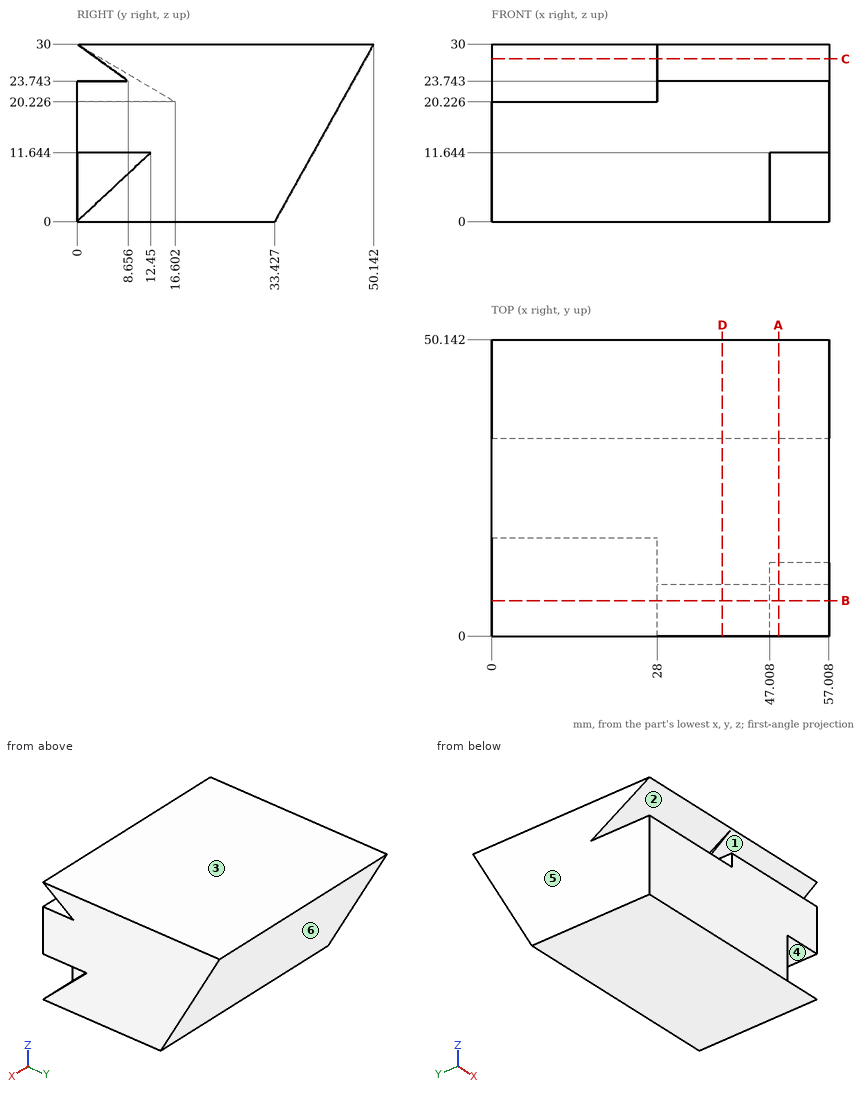
Verification items for this drawing (mm, ordinates from the low corner). A direction names the side the tool comes from. Give positions to 0.01 mm unless a question says otherwise; leave off trailing zeros. Loops run counter-clockwise (first coordinate to the right, second up) from the corner with the lowest first, then second, coordinate; pieces in that order, holes last. Notation, with made-up numbers: M -16.75,28 L 2.25,28 A14 ccw 2.25,42 Z; hole C -11,-10 d7. An arc over 180 degrees is marked long. Return JSON: item names as keys, results as strings. Group by question number.
1. Cross-section at A-A on x = 48.5. Record the boundary of the cut face in (y, z).
2. Tool access check on the marked faces 1, 2 and 3. Record the directions out of +Z, -Z, +X, -X, +Y, -Y that give a thin tool (end or side, any length) a straight path to the whole face; none if there is none.
3. Thickness scan on L1, parallel to Z at x = 8, y = 8.5 (1 decimal); L2, parallel to X at y = 10, z = 11.5; L3, parallel to Z at x = 5.5, y = 10.5 (1 decimal). Record the ranges inside material, lowest first.
4. Cross-section at D-D on x = 39. Record the boundary of the cut face in (y, z), plus the area to 3 significant figures.
5. Cross-section at C-C on z = 27.5. Record the boundary of the cut face in (x, y), plus the area to 3 significant figures.
6. Mould release check, pull along Z, two halves, no side actions. Record for the marked faces 4, 5 and 6: released by +Z, released by -Z, zero draft, split by the parting line, or undercut.
7. Cross-section at B-B on y = 6. Record the boundary of the cut face in (x, z) (1 decimal), plus the area to 3 significant figures.
8. Go/stop test with flat-tipped pins: pin 1 (1 mm diameter, centred on x = 39, z = 18, fed in from +Y) (1 decimal); pin 2 (2 mm diameter, centred on x = 15, z = 8, fed in from +Y); pin 3 (2 mm diameter, centred on x = 6, z = 9, fed in from +Y). Record where each tip stops, or that it passes through.
Return value:
{
 "1": {"outline": "M 0,0 L 33.43,0 L 50.14,30 L 0,30 L 8.66,23.74 L 0,23.74 L 0,11.64 L 12.45,11.64 Z"},
 "2": {"face 1": "+X, -X, -Y", "face 2": "-X, -Y", "face 3": "+Z, +X, -X, +Y, -Y"},
 "3": {"L1": "0 to 20.2, 25 to 30", "L2": "0 to 47.01", "L3": "0 to 20.2, 23.8 to 30"},
 "4": {"outline": "M 0,0 L 33.43,0 L 50.14,30 L 0,30 L 8.66,23.74 L 0,23.74 Z", "area": "1,230 mm^2"},
 "5": {"outline": "M 0,4.25 L 28,4.25 L 28,3.46 L 57.01,3.46 L 57.01,48.75 L 0,48.75 Z", "area": "2,560 mm^2"},
 "6": {"face 4": "undercut", "face 5": "zero draft", "face 6": "released by -Z"},
 "7": {"outline": "M 0,0 L 57,0 L 57,5.6 L 47,5.6 L 47,11.6 L 57,11.6 L 57,23.7 L 28,23.7 L 28,20.2 L 0,20.2 Z; M 0,26.5 L 28,26.5 L 28,25.7 L 57,25.7 L 57,30 L 0,30 Z", "area": "1,420 mm^2"},
 "8": {"pin 1": "y = 43.7", "pin 2": "y = 38.44", "pin 3": "y = 39"}
}
